Work out the finished part from the listing and answer in its coordinate system (mm). A direction names the side the tool comes from. Coordinates: 2 decimals unless noted, no trailing zeros. Order: outer loops, then holes, each group sorted by start corner. A loop starts at its lowest first (then second) coordinate and runs counter-clockwise, first axis right, second up. Notation, with made-up numbers: (27.5, 14.5) -> (40.5, 14.5) arc R27 cw to (40.5, 40.5) -> close; hole circle Ø5 at (46, 68). An arc over 180 degrees is marked (long way). Write item = value, one per line. Start each with the question number.
Q1. The part is cut by section B-B, the plane y = 14. Determine the outline of the cut face in (x, z).
Q2. The part is cut by section C-C, the plane y = 3.6. Determine the outline of the cut face in (x, z).
Q3. Straight lines are drawn through the part: L1, parallel to Y at x = -1, z = 0.75; L2, parallel to Y at x = -2.5, z = -2; L3, parallel to Z at x = -1.75, y = 15. For each, find the intervals that lie inside material, in ascending order. Write a range as from..to.
Q4. Which of the six approach directions +Z, -Z, +X, -X, +Y, -Y give full straight-line access (tool end or side, diameter ignored) to faces 1 (the cylindrical face through (-1.05, 4.82, -3.34)), 2 (the cylindrical face through (-0.77, 4.54, -2.35)), 3 (the conical face through (2.18, 29.96, 2.23)), 4 (the cylindrical face through (2.14, 26.69, -2.1))?
Q5. For a pull along Y with two mould halves and no side action, classify faces 5 (the flat face through (0, 8.8, 0)), 6 (the flat face through (2.834, 11.923, -0.004)), 7 (the conical face through (-1.961, 30.892, -2.005)), 8 (the flat face through (-0.004, 11.624, 2.856)) as +Y half, -Y half, draft (parallel to the pull), parting line (faces both ways), or undercut.
Q6. Flat-ended cylindrical pins translate along their axes: pin 1 (3 mm diameter, centred on x = -0.5, y = 22, fed in from -Z); pin 2 (2 mm diameter, centred on x = 2.5, y = 4, fed in from +Z); pin 3 (0.6 mm diameter, centred on x = 2.5, y = 12, fed in from -Z). Find the tip coordinate at first contact, or state that the pin passes through.
Q7. The part is cut by section A-A, the plane y = 19. Determine the outline of the cut face in (x, z), plus the area to 3 significant figures.
```python
from build123d import *
from OCP.BRepFilletAPI import BRepFilletAPI_MakeChamfer

# Parameters (mm, degrees)
SKETCH1_W               = 3.5
SKETCH1_H               = 9.5
SKETCH2_R               = 2.2
CUT_EXTRUDE1_DEPTH      = 19.4
SKETCH3_R               = 2
CUT_EXTRUDE2_DEPTH      = 8.8
CUT_EXTRUDE3_DEPTH      = 32.972644557
CUT_EXTRUDE4_DEPTH      = 32.972644557
CUT_EXTRUDE5_DEPTH      = 0.3
CUT_EXTRUDE5_DEPTH_BACK = 0.3
CUT_EXTRUDE6_DEPTH      = 0.3
CUT_EXTRUDE6_DEPTH_BACK = 0.3
CUT_EXTRUDE7_START      = 5.3
SKETCH15_R              = 3.5
SKETCH15_R_2            = 3
CUT_EXTRUDE7_DEPTH      = 5.3
CHAMFER1_SIZE           = 0.4
CHAMFER1_SIZE2          = 0.407653471


# Read off the part's stored shape, not the designer's step: CSK for M3 Oval Head Machine Screw1
with BuildPart() as part:
    # Sketch1 → Revolve1 (revolve)
    with BuildSketch(Plane.XY, mode=Mode.PRIVATE) as revolve1_sk:
        Polygon((0, 9.5), (3.5, 9.5), (3.1, 31), (0, 31), align=None)
        with Locations((1.75, 4.75)):
            Rectangle(SKETCH1_W, SKETCH1_H)
    revolve(revolve1_sk.sketch.rotate(Axis((0, 0, 0), (0, 1, 0)), 90), axis=Axis((0, 0, 0), (0, 1, 0)))

    # Sketch2 → Cut-Extrude1 (cut)
    with BuildSketch(Plane(origin=(0, 31, 0), x_dir=(1, 0, 0), z_dir=(0, 1, 0))):
        with Locations(Location((0, 0, 0), (0, 0, 270))):
            Circle(SKETCH2_R)
    extrude(amount=-CUT_EXTRUDE1_DEPTH, mode=Mode.SUBTRACT)

    # Sketch3 → Cut-Extrude2 (cut)
    with BuildSketch(Plane.XZ):
        with Locations(Location((0, -0.502631205, 0), (0, 0, 270))):
            Circle(SKETCH3_R)
    extrude(amount=-CUT_EXTRUDE2_DEPTH, mode=Mode.SUBTRACT)

    # Sketch5 → Cut-Extrude3 (cut, through all)
    with BuildSketch(Plane(origin=(3.5, 0, 0), x_dir=(0, 0, -1), z_dir=(1, 0, 0))):
        Polygon((0.3, 13.5), (-0.3, 13.5), (-0.005, 31), (0.005, 31), align=None)
    extrude(amount=-CUT_EXTRUDE3_DEPTH, mode=Mode.SUBTRACT)

    # Sketch9 → Cut-Extrude4 (cut, through all)
    with BuildSketch(Plane.XY.offset(3.5)):
        Polygon((0.3, 13.5), (-0.3, 13.5), (-0.005, 31), (0.005, 31), align=None)
    extrude(amount=-CUT_EXTRUDE4_DEPTH, mode=Mode.SUBTRACT)

    # Sketch11 → Cut-Extrude5 (cut, two sides: drawn at the far end of the back side and taken through both)
    with BuildSketch(Plane.XY.offset(-CUT_EXTRUDE5_DEPTH_BACK)):
        Polygon((-3.485105978, 10.300553669), (-3.425581395, 13.5), (-2.2, 13.5), align=None)
        Polygon((2.2, 13.5), (3.485105978, 10.300553669), (3.425581395, 13.5), align=None)
    extrude(amount=CUT_EXTRUDE5_DEPTH + CUT_EXTRUDE5_DEPTH_BACK, mode=Mode.SUBTRACT)

    # Sketch14 → Cut-Extrude6 (cut, two sides: drawn at the far end of the back side and taken through both)
    with BuildSketch(Plane(origin=(0, 0, 0), x_dir=(0, 0, -1), z_dir=(1, 0, 0)).offset(-CUT_EXTRUDE6_DEPTH_BACK)):
        Polygon((2.2, 13.5), (3.425581395, 13.5), (3.494418605, 9.8), align=None)
        Polygon((-3.425581395, 13.5), (-3.494418605, 9.8), (-2.2, 13.5), align=None)
    extrude(amount=CUT_EXTRUDE6_DEPTH + CUT_EXTRUDE6_DEPTH_BACK, mode=Mode.SUBTRACT)

    # Sketch15 → Cut-Extrude7 (cut)
    with BuildSketch(Plane(origin=(0, 24, 0), x_dir=(1, 0, 0), z_dir=(0, 1, 0)).offset(CUT_EXTRUDE7_START)):
        with Locations(Location((0, 0, 0), (0, 0, 90))):
            Circle(SKETCH15_R)
        Circle(SKETCH15_R_2, mode=Mode.SUBTRACT)
    extrude(amount=-CUT_EXTRUDE7_DEPTH, mode=Mode.SUBTRACT)

    # CSK for M3 Oval Head Machine Screw1 outl → CSK for M3 Oval Head Machine Screw1 (revolve, cut)
    with BuildSketch(Plane.XZ.offset(-3.6)):
        Polygon((0, 0.819848747), (1.5, 0.819848747), (1.5, 2.75), (2.250138013, 3.500138013), (0, 3.500138013), align=None)
    revolve(axis=Axis((0, 3.6, 0), (0, 0, 1)), mode=Mode.SUBTRACT)

    # Chamfer1: one chamfer whose edges measure the first distance from different faces: ONE call of the kernel's chamfer builder (chamfer() names one face for all edges)
    chamfer1_edges_1 = [part.edges().sort_by_distance(p)[0] for p in [
        (-2.192031022, 31, -2.192031022),
    ]]
    chamfer1_side_1 = [part.faces().sort_by_distance(p)[0] for p in [
        (-2.203213175, 30.15, -2.203213175),
    ]]
    chamfer1_edges_2 = [part.edges().sort_by_distance(p)[0] for p in [
        (2.192031022, 31, -2.192031022),
    ]]
    chamfer1_side_2 = [part.faces().sort_by_distance(p)[0] for p in [
        (2.203213175, 30.15, -2.203213175),
    ]]
    chamfer1_edges_3 = [part.edges().sort_by_distance(p)[0] for p in [
        (2.192031022, 31, 2.192031022),
    ]]
    chamfer1_side_3 = [part.faces().sort_by_distance(p)[0] for p in [
        (2.203213175, 30.15, 2.203213175),
    ]]
    chamfer1_edges_4 = [part.edges().sort_by_distance(p)[0] for p in [
        (-2.192031022, 31, 2.192031022),
    ]]
    chamfer1_side_4 = [part.faces().sort_by_distance(p)[0] for p in [
        (-2.203213175, 30.15, 2.203213175),
    ]]
    chamfer1_edges_5 = [part.edges().sort_by_distance(p)[0] for p in [
        (-1.555634919, 31, -1.555634919),
        (1.555634919, 31, -1.555634919),
        (1.555634919, 31, 1.555634919),
        (-1.555634919, 31, 1.555634919),
        (0, 0, 1.497368795),
    ]]
    chamfer1 = BRepFilletAPI_MakeChamfer(part.part.solid().wrapped)
    for e in chamfer1_edges_1:
        chamfer1.Add(CHAMFER1_SIZE, CHAMFER1_SIZE2, e.wrapped, chamfer1_side_1[0].wrapped)  # the first distance lies on this face
    for e in chamfer1_edges_2:
        chamfer1.Add(CHAMFER1_SIZE, CHAMFER1_SIZE2, e.wrapped, chamfer1_side_2[0].wrapped)  # the first distance lies on this face
    for e in chamfer1_edges_3:
        chamfer1.Add(CHAMFER1_SIZE, CHAMFER1_SIZE2, e.wrapped, chamfer1_side_3[0].wrapped)  # the first distance lies on this face
    for e in chamfer1_edges_4:
        chamfer1.Add(CHAMFER1_SIZE, CHAMFER1_SIZE2, e.wrapped, chamfer1_side_4[0].wrapped)  # the first distance lies on this face
    for e in chamfer1_edges_5:
        chamfer1.Add(CHAMFER1_SIZE, e.wrapped)
    add(Compound.cast(chamfer1.Shape()), mode=Mode.REPLACE)


solid = part.part
```
Model answer:
q1.outline = (-3.4, -0.29) arc R3.42 ccw to (-0.29, -3.4) -> (-0.29, -2.18) arc R2.2 cw to (-2.18, -0.29) -> close; (-3.4, 0.29) -> (-2.18, 0.29) arc R2.2 cw to (-0.29, 2.18) -> (-0.29, 3.4) arc R3.42 ccw to start; (0.29, -3.4) arc R3.42 ccw to (3.4, -0.29) -> (2.18, -0.29) arc R2.2 cw to (0.29, -2.18) -> close; (0.29, 2.18) arc R2.2 cw to (2.18, 0.29) -> (3.4, 0.29) arc R3.42 ccw to (0.29, 3.4) -> close
q2.outline = (-1.77, 3.02) arc R3.5 ccw (long way) to (1.77, 3.02) -> (1.5, 2.75) -> (1.5, 0.82) arc R2 cw (long way) to (-1.5, 0.82) -> (-1.5, 2.75) -> close
q3.L1 = 8.8..11.6
q3.L2 = 0..24
q3.L3 = -2.91..-1.33, 1.33..2.91
q4.face_1 = +Y, -Y
q4.face_2 = -Y
q4.face_3 = +Z, +X, +Y
q4.face_4 = -Z, +X
q5.face_5 = -Y half
q5.face_6 = undercut
q5.face_7 = +Y half
q5.face_8 = undercut
q6.pin_1 = -3.29
q6.pin_2 = 3.1
q6.pin_3 = -2.66
q7.outline = (-3.32, -0.21) arc R3.32 ccw to (-0.21, -3.32) -> (-0.21, -2.19) arc R2.2 cw to (-2.19, -0.21) -> close; (-3.32, 0.21) -> (-2.19, 0.21) arc R2.2 cw to (-0.21, 2.19) -> (-0.21, 3.32) arc R3.32 ccw to start; (0.21, -3.32) arc R3.32 ccw to (3.32, -0.21) -> (2.19, -0.21) arc R2.2 cw to (0.21, -2.19) -> close; (0.21, 2.19) arc R2.2 cw to (2.19, 0.21) -> (3.32, 0.21) arc R3.32 ccw to (0.21, 3.32) -> close
q7.area = 17.6 mm2
